```python
from build123d import *

# Parameters (mm, degrees)
SKETCH1_R           = 43.053
SKETCH1_R_2         = 39.37
BOSS_EXTRUDE1_DEPTH = 4.318
SKETCH2_W           = 2.54
SKETCH2_H           = 4.749764311
CUT_EXTRUDE1_DEPTH  = 62.039059151


with BuildPart() as part:
    # Sketch1 → Boss-Extrude1 (new body)
    with BuildSketch(Plane.XY):
        Circle(SKETCH1_R)
        Circle(SKETCH1_R_2, mode=Mode.SUBTRACT)
    extrude(amount=BOSS_EXTRUDE1_DEPTH)

    # Sketch2 → Cut-Extrude1 (cut, through all)
    with BuildSketch(Plane.XY):
        with Locations((0, -41.724392952)):
            Rectangle(SKETCH2_W, SKETCH2_H)
    extrude(amount=CUT_EXTRUDE1_DEPTH, mode=Mode.SUBTRACT)


solid = part.part
```
The listing builds one solid part. Answer for the finished solid, in the listing's coordinates (mm). A direction names the side the tool comes from. Coordinates: 2 decimals unless noted, no trailing zeros. Loops run counter-clockwise (first coordinate to the right, second up) from the corner with the lowest first, then second, coordinate; pieces in that order, holes last. Notation, with made-up numbers: M 41.25,4.5 L 56.25,4.5 A24 ccw 56.25,21.5 Z; hole C -3.5,-25.75 d7. An arc over 180 degrees is marked long. Answer as a JSON object with one key per item and string values. Group by question number.
Item 1: Section D-D (x = 0) is taken. Write down the section's boundary in (y, z), and give its area (3 significant figures).
Item 2: Section A-A (x = 33) is taken. Write down the section's boundary in (y, z), and give its area (3 significant figures).
Item 3: Consider L1, parallel to X at y = 0, z = 1.5; L2, parallel to Y at x = -5.5, z = 1.3; L3, parallel to Y at x = 14, z = 3.2. Determine where each line is inside the solid, lowest interval first.
Item 4: Which of the six approach directions +Z, -Z, +X, -X, +Y, -Y give full straight-line access (tool end or side, diameter ignored) to faces 3 (the face through (1.27, -41, 2)), 4 (the face through (9.4, 38.5, 4.318))?
Item 5: Section B-B (y = -31) is taken. Write down the section's boundary in (x, z), and give its area (3 significant figures).
Item 6: Each of these flat-tipped pins is pushed along its axis until it touches: P1, Ø1, axis at x = -6.5, z = 2, coming from the +Y side; P2, Ø2, axis at x = -3.5, z = 3, coming from the -Y side; P3, Ø1.5, axis at y = -27.5, z = 1.5, coming from the +X side. Where does it stop, or does it pass through?
Item 7: Section C-C (z = 3.25) is taken. Write down the section's boundary in (x, y), and give its area (3 significant figures).
Item 8: Determine the mould class of faces 1 (the face through (9.4, 38.5, 0)), 2 (the face through (-1.27, -41, 2)) for opening direction X: +X half, -X half, draft (parallel to the pull), parting line (faces both ways), or undercut.
Solved:
{
 "1": {"outline": "M 39.37,0 L 43.05,0 L 43.05,4.32 L 39.37,4.32 Z", "area": "15.9 mm2"},
 "2": {"outline": "M -27.65,0 L -21.47,0 L -21.47,4.32 L -27.65,4.32 Z; M 21.47,0 L 27.65,0 L 27.65,4.32 L 21.47,4.32 Z", "area": "53.4 mm2"},
 "3": {"L1": "x = -43.05 to -39.37, 39.37 to 43.05", "L2": "y = -42.7 to -38.98, 38.98 to 42.7", "L3": "y = -40.71 to -36.8, 36.8 to 40.71"},
 "4": {"face 3": "+Z, -Z, -Y", "face 4": "+Z, +X, -X, +Y, -Y"},
 "5": {"outline": "M -29.88,0 L -24.27,0 L -24.27,4.32 L -29.88,4.32 Z; M 24.27,0 L 29.88,0 L 29.88,4.32 L 24.27,4.32 Z", "area": "48.4 mm2"},
 "6": {"P1": "stops at y = 42.63", "P2": "stops at y = -42.98", "P3": "stops at x = 33.73"},
 "7": {"outline": "M -1.27,-43.03 L -1.27,-39.35 A39.37 cw long 1.27,-39.35 L 1.27,-43.03 A43.05 ccw long Z", "area": "944 mm2"},
 "8": {"face 1": "draft", "face 2": "undercut"}
}
